```python
from build123d import *

# Parameters (mm, degrees)
F1_R     = 16.55
F0_DEPTH = 25


with BuildPart() as f0:
    # F1 (on Front) → F0 (new body)
    with BuildSketch(Plane.XZ):
        with BuildLine():
            ThreePointArc((18.9471511403, -1.9768570177), (19.0242704094, -0.9897653202), (19.05, 0))
            ThreePointArc((19.05, 0), (17.0081092666, 8.5806013294), (11.3201607165, 15.3217643028))
            ThreePointArc((11.3201607165, 15.3217643028), (3.1862146863, 18.7816542395), (-5.6337146577, 18.1979053508))
            ThreePointArc((-5.6337146577, 18.1979053508), (-12.7048225923, 14.1947167248), (-17.4644289069, 7.6089567588))
            ThreePointArc((-17.4644289069, 7.6089567588), (-18.9951016681, 1.4452033137), (-18.4145629505, -4.8791773224))
            ThreePointArc((-18.4145629505, -4.8791773224), (1.4753909085, -18.9927807776), (18.9471511403, -1.9768570177))
        make_face()
        Circle(F1_R, mode=Mode.SUBTRACT)
        with BuildLine():
            ThreePointArc((11.3201607165, 15.3217643028), (17.0081092666, 8.5806013294), (19.05, 0))
            ThreePointArc((19.05, 0), (19.0242704094, -0.9897653202), (18.9471511403, -1.9768570177))
            Line((18.9471511403, -1.9768570177), (367.068516355, 422.1730984288))
            Line((367.068516355, 422.1730984288), (358.5591705204, 445.5523339637))
            Line((358.5591705204, 445.5523339637), (354.4296862364, 456.8979987878))
            Line((354.4296862364, 456.8979987878), (197.6336692676, 265.8582343353))
            Line((197.6336692676, 265.8582343353), (68.718206586, 108.788047853))
            Line((68.718206586, 108.788047853), (6.5665120874, 33.0626225082))
            Line((6.5665120874, 33.0626225082), (11.3201607165, 15.3217643028))
        make_face()
        with BuildLine():
            ThreePointArc((-5.6337146577, 18.1979053508), (3.1862146863, 18.7816542395), (11.3201607165, 15.3217643028))
            Line((11.3201607165, 15.3217643028), (6.5665120874, 33.0626225082))
            Line((6.5665120874, 33.0626225082), (-36.9494436056, 195.4663800944))
            Line((-36.9494436056, 195.4663800944), (-44.0597309982, 222.0023338999))
            Line((-44.0597309982, 222.0023338999), (-104.6644659355, 448.182283865))
            Line((-104.6644659355, 448.182283865), (-133.4490555589, 440.4694763209))
            Line((-133.4490555589, 440.4694763209), (-124.5620482674, 407.302713582))
            Line((-124.5620482674, 407.302713582), (-121.5848978652, 396.1918370193))
            Line((-121.5848978652, 396.1918370193), (-18.4742653371, 11.3777176238))
            Line((-18.4742653371, 11.3777176238), (-17.4644289069, 7.6089567588))
            ThreePointArc((-17.4644289069, 7.6089567588), (-12.7048225923, 14.1947167248), (-5.6337146577, 18.1979053508))
        make_face()
        with BuildLine():
            Line((-72.3879589454, 4.6290750499), (-18.4145629505, -4.8791773224))
            ThreePointArc((-18.4145629505, -4.8791773224), (-18.9951016681, 1.4452033137), (-17.4644289069, 7.6089567588))
            Line((-17.4644289069, 7.6089567588), (-18.4742653371, 11.3777176238))
            Line((-18.4742653371, 11.3777176238), (-69.612055331, 20.3864339378))
            ThreePointArc((-69.612055331, 20.3864339378), (-70.9081149957, 12.4915662651), (-72.3879589454, 4.6290750499))
        make_face()
        Polygon((358.5591705204, 445.5523339637), (367.068516355, 422.1730984288), (370.4887177882, 412.7761722209), (387.4031849624, 418.9325348008), (404.3176521365, 425.0888973806), (391.2308402699, 461.0446174767), (364.9853356541, 533.153548771), (331.1564013058, 520.8408236113), (334.576602739, 511.4438974034), (343.6802788522, 486.4317528486), (354.4296862364, 456.8979987878), align=None)
        Polygon((-44.0597309982, 222.0023338999), (-36.9494436056, 195.4663800944), (128.9154626816, 322.2587492585), (343.6802788522, 486.4317528486), (334.576602739, 511.4438974034), align=None)
        with BuildLine():
            Line((-103.9121348451, 10.1825484742), (-72.3879589454, 4.6290750499))
            ThreePointArc((-72.3879589454, 4.6290750499), (-70.9081149957, 12.4915662651), (-69.612055331, 20.3864339378))
            Line((-69.612055331, 20.3864339378), (-101.1362312306, 25.9399073622))
            ThreePointArc((-101.1362312306, 25.9399073622), (-102.4228327716, 18.043373494), (-103.9121348451, 10.1825484742))
        make_face()
        with BuildLine():
            Line((-124.5620482674, 407.302713582), (-187.7531740158, 334.3521096451))
            ThreePointArc((-187.7531740158, 334.3521096451), (-184.1317567279, 331.2589177075), (-180.5536370153, 328.1157411523))
            Line((-180.5536370153, 328.1157411523), (-121.5848978652, 396.1918370193))
            Line((-121.5848978652, 396.1918370193), (-124.5620482674, 407.302713582))
        make_face()
        with BuildLine():
            ThreePointArc((-180.5536370153, 328.1157411523), (-184.1317567279, 331.2589177075), (-187.7531740158, 334.3521096451))
            Line((-187.7531740158, 334.3521096451), (-208.7069809814, 310.1621169077))
            ThreePointArc((-208.7069809814, 310.1621169077), (-205.0833359165, 307.0714968135), (-201.5074439809, 303.9257484149))
            Line((-201.5074439809, 303.9257484149), (-180.5536370153, 328.1157411523))
        make_face()
        with BuildLine():
            Line((-400.6354173431, 62.4549653328), (-103.9121348451, 10.1825484742))
            ThreePointArc((-103.9121348451, 10.1825484742), (-102.4228327716, 18.043373494), (-101.1362312306, 25.9399073622))
            Line((-101.1362312306, 25.9399073622), (-397.1350282031, 78.084694838))
            Line((-397.1350282031, 78.084694838), (-201.5074439809, 303.9257484149))
            ThreePointArc((-201.5074439809, 303.9257484149), (-205.0833359165, 307.0714968135), (-208.7069809814, 310.1621169077))
            Line((-208.7069809814, 310.1621169077), (-404.7393478146, 83.8537645513))
            ThreePointArc((-404.7393478146, 83.8537645513), (-398.5615625862, 79.3027613179), (-396.2064961559, 72))
            ThreePointArc((-396.2064961559, 72), (-397.3676583592, 66.7387494433), (-400.6354173431, 62.4549653328))
        make_face()
        with BuildLine():
            ThreePointArc((-404.7393478146, 83.8537645513), (-420.9827692162, 69.6456169071), (-400.6354173431, 62.4549653328))
            ThreePointArc((-400.6354173431, 62.4549653328), (-397.3676583592, 66.7387494433), (-396.2064961559, 72))
            ThreePointArc((-396.2064961559, 72), (-398.5615625862, 79.3027613179), (-404.7393478146, 83.8537645513))
        make_face()
    extrude(amount=F0_DEPTH)


solid = f0.part
```
Model file for the job. Use its own axes, mm. A direction names the side the tool comes from. Round coordinates to 2 decimals unless told otherwise and drop trailing zeros. Write each loop counter-clockwise with the first axis right and the second up, starting at its lowest first coordinate (ties: lowest second). Pieces come first, ordered by that corner, then holes. Notation, with made-up numbers: (-28, -13.5) - (-18, -13.5) arc R15 cw to (-18, 12.5) - close; hole circle Ø6 at (66, 74). An arc over 180 degrees is marked (long way). Use CSV: the item, a comma, the result in double quotes. Start each with the question number.
Item 1: Drill centre lines: L1, parallel to X at y = -8, z = 402.5; L2, parallel to X at y = -15.5, z = 117; L3, parallel to X at y = -4.5, z = 344.5. Where is each one in solid material? Low to high. Write a range as [from, to].
Item 2: Tool access for faces 1 (the face through (-14.887, -12.325, 113.128)), 2 (the face through (20, -25, 258)), 3 (the face through (-129.07, -12.32, 424.12)), 4 (the face through (-73.94, -12.32, 333.51)), 5 (the face through (348.308, -12.325, 527.083)): list every direction of +Z, -Z, +X, -X, +Y, -Y with a clear straight run to the whole face (end or side of a thin tool).
Item 3: Band-saw the part on B-B (z = 236.5). Write the cut outline in (x, y).
Item 4: Pin check, flat tips, straight feed: P1, Ø1, axis at x = -128.5, y = -3.5, coming from the -Z side; P2, Ø12, axis at y = -14, z = 190.5, coming from the +X side; P3, Ø4, axis at x = -265, y = -22, coming from the -Z side. Stop position of each tip, or through.
Item 5: Two-plate mould, pull along X, no slides. Class faces 6 (the face through (-118.86, -12.32, 444.38)), 7 (the face through (-3.588, -12.325, -16.156)), 8 (the face through (1.106, -12.325, -19.018)), 9 (the face through (182.933, -12.325, 247.947)): released by +X, released by -X, zero draft, split by the parting line, or undercut.
Item 6: Band-saw the part on A-A (y = -13.5). Write the cut outline in (x, z).
Item 7: Band-saw the part on C-C (x = 215.5). Write the cut outline in (y, z), and give its area (3 significant figures).
Item 8: Band-saw the part on D-D (x = -304.5). Write the cut outline in (y, z).
Checked values:
1,L1,"x = [-128.72, -92.42], [192.06, 233.88], [309.78, 350.92]"
1,L2,"x = [-376.03, -363.43], [-46.78, -15.92], [75.46, 116.6]"
1,L3,"x = [-178.96, -166.36], [-107.73, -76.88], [116.19, 158.01], [262.18, 303.32]"
2,face 1,"+Y, -Y"
2,face 2,"+Z, -Z, +X, -X, -Y"
2,face 3,"-X, +Y, -Y"
2,face 4,"+Z, +Y, -Y"
2,face 5,"+Z, -X, +Y, -Y"
3,outline,"(-272.51, -25) - (-259.91, -25) - (-259.91, 0) - (-272.51, 0) - close; (-78.8, -25) - (-47.94, -25) - (-47.94, 0) - (-78.8, 0) - close; (-25.09, -25) - (16.73, -25) - (16.73, 0) - (-25.09, 0) - close; (173.54, -25) - (214.68, -25) - (214.68, 0) - (173.54, 0) - close"
4,P1,"stops at z = 14.43"
4,P2,"stops at x = 181.85"
4,P3,"stops at z = 38.21"
5,face 6,"released by -X"
5,face 7,"undercut"
5,face 8,"split by the parting line"
5,face 9,"undercut"
6,outline,"(-404.74, 83.85) arc R12.5 ccw (long way) to (-400.64, 62.45) - (-18.41, -4.88) arc R19.05 ccw to (18.95, -1.98) - (367.07, 422.17) - (370.49, 412.78) - (404.32, 425.09) - (364.99, 533.15) - (331.16, 520.84) - (334.58, 511.44) - (-44.06, 222) - (-104.66, 448.18) - (-133.45, 440.47) - (-124.56, 407.3) - close; hole (-397.14, 78.08) - (-18.47, 11.38) - (-121.58, 396.19) - close; hole (-36.95, 195.47) - (6.57, 33.06) - (354.43, 456.9) - (343.68, 486.43) - close; hole circle Ø33.1 at (0, 0)"
7,outline,"(-25, 237.5) - (0, 237.5) - (0, 287.63) - (-25, 287.63) - close; (-25, 388.45) - (0, 388.45) - (0, 420.42) - (-25, 420.42) - close"
7,area,"2,050 mm²"
8,outline,"(-25, 45.52) - (0, 45.52) - (0, 61.77) - (-25, 61.77) - close; (-25, 185.03) - (0, 185.03) - (0, 199.57) - (-25, 199.57) - close"
